from build123d import *

# Parameters (mm, degrees)
SKETCH1_W                                       = 75
SKETCH1_H                                       = 108
BOSS_EXTRUDE1_DEPTH                             = 10
SKETCH2_R                                       = 6
SKETCH2_R_2                                     = 5
CUT_EXTRUDE2_DEPTH                              = 115.761709642
HOLE_WIZARD_M31_D                               = 3.2
HOLE_WIZARD_M31_CSINK_D                         = 6.3
HOLE_WIZARD_M31_CSINK_ANGLE                     = 90
BOSS_EXTRUDE2_DEPTH                             = 75
BOSS_EXTRUDE3_DEPTH                             = 7
CHAMFER2_SIZE                                   = 0.5
HOLE_WIZARD_M41_DEPTH                           = 10
CHAMFER4_SIZE                                   = 0.5
CUT_EXTRUDE3_DEPTH                              = 122.762603454
CSK_FOR_M2_FLAT_HEAD_MACHINE_SCREW1_D           = 2.2
CSK_FOR_M2_FLAT_HEAD_MACHINE_SCREW1_CSINK_D     = 4.4
CSK_FOR_M2_FLAT_HEAD_MACHINE_SCREW1_CSINK_ANGLE = 90
M5X0_8_TAPPED_HOLE1_D                           = 4.2
M5X0_8_TAPPED_HOLE1_DEPTH                       = 10.4
M5X0_8_TAPPED_HOLE1_TIP                         = 1.2618073
CHAMFER6_SIZE                                   = 10


with BuildPart() as part:
    # Sketch1 → Boss-Extrude1 (new body)
    with BuildSketch(Plane.XY):
        with Locations((0, -54)):
            Rectangle(SKETCH1_W, SKETCH1_H)
    extrude(amount=BOSS_EXTRUDE1_DEPTH)

    # Sketch2 → Cut-Extrude2 (cut, through all)
    with BuildSketch(Plane.XY):
        with Locations((16, -25)):
            Circle(SKETCH2_R)
        with Locations((-17, -25)):
            Circle(SKETCH2_R_2)
    extrude(amount=CUT_EXTRUDE2_DEPTH, mode=Mode.SUBTRACT)

    # Зенковка для  винта с плоской головкой M31 (through all)
    with Locations(Plane.XY.offset(10)):
        with Locations((26.825317547, -18.75), (5.174682453, -18.75), (5.174682453, -31.25), (26.825317547, -31.25)):
            CounterSinkHole(HOLE_WIZARD_M31_D / 2, HOLE_WIZARD_M31_CSINK_D / 2, counter_sink_angle=HOLE_WIZARD_M31_CSINK_ANGLE)

    # Sketch13 → Boss-Extrude2 (add, through all)
    with BuildSketch(Plane(origin=(37.5, 0, 0), x_dir=(0, 0, -1), z_dir=(1, 0, 0))):
        Polygon((-10, -97.69), (-13.96, -101.65), (-13.96, -108), (-10, -108), (0, -108), (3.96, -108), (3.96, -101.65), (0, -97.69), align=None)
    extrude(amount=-BOSS_EXTRUDE2_DEPTH)

    # Sketch14 → Boss-Extrude3 (add)
    with BuildSketch(Plane.XZ.offset(108)):
        with BuildLine():
            Line((-2.5, 0), (-2.5, 10))
            ThreePointArc((-2.5, 10), (0, 12.5), (2.5, 10))
            Line((2.5, 10), (2.5, 0))
            ThreePointArc((2.5, 0), (0, -2.5), (-2.5, 0))
        make_face()
        with BuildLine():
            Line((22.5, 0), (22.5, 10))
            ThreePointArc((22.5, 10), (25, 12.5), (27.5, 10))
            Line((27.5, 10), (27.5, 0))
            ThreePointArc((27.5, 0), (25, -2.5), (22.5, 0))
        make_face()
        with BuildLine():
            Line((-27.5, 0), (-27.5, 10))
            ThreePointArc((-27.5, 10), (-25, 12.5), (-22.5, 10))
            Line((-22.5, 10), (-22.5, 0))
            ThreePointArc((-22.5, 0), (-25, -2.5), (-27.5, 0))
        make_face()
    extrude(amount=BOSS_EXTRUDE3_DEPTH)

    # Chamfer2
    chamfer2_edges = [part.edges().sort_by_distance(p)[0] for p in [
        (-25, -115, 12.5),
        (-27.5, -115, 5),
        (-25, -115, -2.5),
        (-22.5, -115, 5),
        (0, -115, 12.5),
        (-2.5, -115, 5),
        (0, -115, -2.5),
        (2.5, -115, 5),
        (25, -115, 12.5),
        (22.5, -115, 5),
        (25, -115, -2.5),
        (27.5, -115, 5),
    ]]
    chamfer(chamfer2_edges, length=CHAMFER2_SIZE)

    # Зенковка для  винта с потайной головкой с внутренним шестигранником M41: read off the stored shape, not the designer's step
    # Зенковка для  винта с потайной головкой с внутренним шестигранником M41 outline → Зенковка для  винта с потайной головкой с внутренним шестигранником M41 (cut)
    with BuildSketch(Plane.XY):
        with BuildLine():
            Line((13.75, -36.25), (13.75, -38.75))
            ThreePointArc((13.75, -38.75), (16, -41), (18.25, -38.75))
            Line((18.25, -38.75), (18.25, -36.25))
            ThreePointArc((18.25, -36.25), (16, -34), (13.75, -36.25))
        make_face()
        with BuildLine():
            Line((18.25, -13.75), (18.25, -11.25))
            ThreePointArc((18.25, -11.25), (16, -9), (13.75, -11.25))
            Line((13.75, -11.25), (13.75, -13.75))
            ThreePointArc((13.75, -13.75), (16, -16), (18.25, -13.75))
        make_face()
    extrude(amount=HOLE_WIZARD_M41_DEPTH, mode=Mode.SUBTRACT)

    # Hole Wizard M41 2: loft between two sections, ruled curve by curve
    hole_wizard_m41_2_from = [
        Edge.make_three_point_arc((13.75, -38.75, 7.77), (14.409009742, -40.340990258, 7.77), (16, -41, 7.77)),
        Edge.make_three_point_arc((16, -41, 7.77), (17.590990258, -40.340990258, 7.77), (18.25, -38.75, 7.77)),
        Edge.make_three_point_arc((18.25, -36.25, 7.77), (17.590990258, -34.659009742, 7.77), (16, -34, 7.77)),
        Edge.make_three_point_arc((16, -34, 7.77), (14.409009742, -34.659009742, 7.77), (13.75, -36.25, 7.77)),
        Edge.make_line((18.25, -38.75, 7.77), (18.25, -36.25, 7.77)),
        Edge.make_line((13.75, -38.75, 7.77), (13.75, -36.25, 7.77)),
    ]
    hole_wizard_m41_2_to = [
        Edge.make_three_point_arc((11.52, -38.75, 10), (12.83216162, -41.91783838, 10), (16, -43.23, 10)),
        Edge.make_three_point_arc((16, -43.23, 10), (19.16783838, -41.91783838, 10), (20.48, -38.75, 10)),
        Edge.make_three_point_arc((20.48, -36.25, 10), (19.16783838, -33.08216162, 10), (16, -31.77, 10)),
        Edge.make_three_point_arc((16, -31.77, 10), (12.83216162, -33.08216162, 10), (11.52, -36.25, 10)),
        Edge.make_line((20.48, -38.75, 10), (20.48, -36.25, 10)),
        Edge.make_line((11.52, -38.75, 10), (11.52, -36.25, 10)),
    ]
    hole_wizard_m41_2 = Solid(Shell([*[Face.make_surface_from_curves(hole_wizard_m41_2_from[k], hole_wizard_m41_2_to[k]) for k in range(6)], Face(Wire(hole_wizard_m41_2_from)), Face(Wire(hole_wizard_m41_2_to))]))
    add(hole_wizard_m41_2, mode=Mode.SUBTRACT)

    # Hole Wizard M41 3: loft between two sections, ruled curve by curve
    hole_wizard_m41_3_from = [
        Edge.make_three_point_arc((13.75, -13.75, 7.77), (14.409009742, -15.340990258, 7.77), (16, -16, 7.77)),
        Edge.make_three_point_arc((16, -16, 7.77), (17.590990258, -15.340990258, 7.77), (18.25, -13.75, 7.77)),
        Edge.make_three_point_arc((18.25, -11.25, 7.77), (17.590990258, -9.659009742, 7.77), (16, -9, 7.77)),
        Edge.make_three_point_arc((16, -9, 7.77), (14.409009742, -9.659009742, 7.77), (13.75, -11.25, 7.77)),
        Edge.make_line((18.25, -13.75, 7.77), (18.25, -11.25, 7.77)),
        Edge.make_line((13.75, -13.75, 7.77), (13.75, -11.25, 7.77)),
    ]
    hole_wizard_m41_3_to = [
        Edge.make_three_point_arc((11.52, -13.75, 10), (12.83216162, -16.91783838, 10), (16, -18.23, 10)),
        Edge.make_three_point_arc((16, -18.23, 10), (19.16783838, -16.91783838, 10), (20.48, -13.75, 10)),
        Edge.make_three_point_arc((20.48, -11.25, 10), (19.16783838, -8.08216162, 10), (16, -6.77, 10)),
        Edge.make_three_point_arc((16, -6.77, 10), (12.83216162, -8.08216162, 10), (11.52, -11.25, 10)),
        Edge.make_line((20.48, -13.75, 10), (20.48, -11.25, 10)),
        Edge.make_line((11.52, -13.75, 10), (11.52, -11.25, 10)),
    ]
    hole_wizard_m41_3 = Solid(Shell([*[Face.make_surface_from_curves(hole_wizard_m41_3_from[k], hole_wizard_m41_3_to[k]) for k in range(6)], Face(Wire(hole_wizard_m41_3_from)), Face(Wire(hole_wizard_m41_3_to))]))
    add(hole_wizard_m41_3, mode=Mode.SUBTRACT)

    # Chamfer4
    chamfer4_edges = [part.edges().sort_by_distance(p)[0] for p in [
        (10, -25, 0),
        (10, -25, 10),
        (13.75, -37.5, 0),
        (16, -41, 0),
        (16, -34, 0),
        (18.25, -37.5, 0),
        (16, -9, 0),
        (18.25, -12.5, 0),
        (13.75, -12.5, 0),
        (16, -16, 0),
        (-22, -25, 0),
        (-22, -25, 10),
        (28.425317547, -31.25, 0),
        (6.774682453, -31.25, 0),
        (6.774682453, -18.75, 0),
        (28.425317547, -18.75, 0),
    ]]
    chamfer(chamfer4_edges, length=CHAMFER4_SIZE)

    # Sketch22 → Cut-Extrude3 (cut, through all)
    with BuildSketch(Plane.XY.offset(10)):
        with BuildLine():
            Line((2.5, -96.69), (-2.5, -96.69))
            ThreePointArc((-2.5, -96.69), (-6.035533906, -95.225533906), (-7.5, -91.69))
            Line((-7.5, -91.69), (-7.5, -57.69))
            ThreePointArc((-7.5, -57.69), (-6.035533906, -54.154466094), (-2.5, -52.69))
            Line((-2.5, -52.69), (2.5, -52.69))
            ThreePointArc((2.5, -52.69), (6.035533906, -54.154466094), (7.5, -57.69))
            Line((7.5, -57.69), (7.5, -91.69))
            ThreePointArc((7.5, -91.69), (6.035533906, -95.225533906), (2.5, -96.69))
        make_face()
        with BuildLine():
            Line((-22.5, -96.69), (-27.5, -96.69))
            ThreePointArc((-27.5, -96.69), (-31.035533906, -95.225533906), (-32.5, -91.69))
            Line((-32.5, -91.69), (-32.5, -57.69))
            ThreePointArc((-32.5, -57.69), (-31.035533906, -54.154466094), (-27.5, -52.69))
            Line((-27.5, -52.69), (-22.5, -52.69))
            ThreePointArc((-22.5, -52.69), (-18.964466094, -54.154466094), (-17.5, -57.69))
            Line((-17.5, -57.69), (-17.5, -91.69))
            ThreePointArc((-17.5, -91.69), (-18.964466094, -95.225533906), (-22.5, -96.69))
        make_face()
        with BuildLine():
            Line((27.5, -96.69), (22.5, -96.69))
            ThreePointArc((22.5, -96.69), (18.964466094, -95.225533906), (17.5, -91.69))
            Line((17.5, -91.69), (17.5, -57.69))
            ThreePointArc((17.5, -57.69), (18.964466094, -54.154466094), (22.5, -52.69))
            Line((22.5, -52.69), (27.5, -52.69))
            ThreePointArc((27.5, -52.69), (31.035533906, -54.154466094), (32.5, -57.69))
            Line((32.5, -57.69), (32.5, -91.69))
            ThreePointArc((32.5, -91.69), (31.035533906, -95.225533906), (27.5, -96.69))
        make_face()
    extrude(amount=-CUT_EXTRUDE3_DEPTH, mode=Mode.SUBTRACT)

    # CSK for M2 Flat Head Machine Screw1 (through all)
    with Locations(Plane.XY.offset(10)):
        with Locations((-17, -17.5), (-17, -32.5)):
            CounterSinkHole(CSK_FOR_M2_FLAT_HEAD_MACHINE_SCREW1_D / 2, CSK_FOR_M2_FLAT_HEAD_MACHINE_SCREW1_CSINK_D / 2, counter_sink_angle=CSK_FOR_M2_FLAT_HEAD_MACHINE_SCREW1_CSINK_ANGLE)

    # M5x0.8 Tapped Hole1
    with Locations(Plane(origin=(0, -108, 0), x_dir=(-1, 0, 0), z_dir=(0, -1, 0))):
        with Locations((32.5, -5), (13.75, -5), (-13.75, -5), (-32.5, -5)):
            Hole(M5X0_8_TAPPED_HOLE1_D / 2, depth=M5X0_8_TAPPED_HOLE1_DEPTH)
            with Locations((0, 0, -(M5X0_8_TAPPED_HOLE1_DEPTH + M5X0_8_TAPPED_HOLE1_TIP / 2))):  # 118° drill point
                Cone(0, M5X0_8_TAPPED_HOLE1_D / 2, M5X0_8_TAPPED_HOLE1_TIP, mode=Mode.SUBTRACT)

    # Chamfer6
    chamfer6_edges = [part.edges().sort_by_distance(p)[0] for p in [
        (-37.5, 0, 5),
        (37.5, 0, 5),
    ]]
    chamfer(chamfer6_edges, length=CHAMFER6_SIZE)


solid = part.part
Input: part model. Units: mm. Frame: model coordinates. A direction names the side the tool comes from. Coordinates: 2 decimals unless noted, no trailing zeros. Write each loop counter-clockwise with the first axis right and the second up, starting at its lowest first coordinate (ties: lowest second). Pieces come first, ordered by that corner, then holes. Notation, with made-up numbers: M -27.75,-9 L 20.25,-9 A23 cw 20.25,17 Z; hole C 8.5,52.25 d4. An arc over 180 degrees is marked long. Answer as a JSON object with one key per item and string values. Group by question number.
(1) Contact query for flat-ended pins moving along their axis: P1, Ø3.5, axis at x = -13.75, z = 5, coming from the -Y side; P2, Ø2.5, axis at x = -32.5, z = 5, coming from the -Y side; P3, Ø22.5, axis at x = -7.5, y = -31.5, coming from the -Z side. Output: stop coordinate, or through.
(2) Ray query, line 1 along X through (y, z) = (-25, 5.75); line 2 along X through (y, z) = (-92, 4.75); line 3 along Y through (x, z) = (16, 5.75). Return the intervals inside material, ascending. Write a range as [from, to].
(3) Section C-C on y = -87.5. Output: boundary loops of the cut face in (x, z), plus the area to 3 significant figures.
(4) Mould query, pull axis Y, two halves, no side actions, for faces 1 (the face through (17.5, -75, 5)), 2 (the face through (-27.5, -111, 5)), 3 (the face through (19, -95.26, 5.07)), 4 (the face through (-24.953, -114.865, -2.135)). Classes: pulls with the +Y half, pulls with the -Y half, needs draft (parallel to the pull), parting line crosses it, or undercut.
(5) Section B-B on x = 0. Output: boundary loops of the cut face in (y, z).
(6) Section A-A on y = -25. Output: boundary loops of the cut face in (x, z), plus the area to 3 significant figures.
(7) Set-up query: faces 5 (the face through (1, -105, -3.96)), 6 (the face through (-1, -48, 10)), 7 (the face through (25, -52.69, 5)), 8 (the face through (24.9, -111.2, 12.5)). Return all of +Z, -Z, +X, -X, +Y, -Y with unobstructed straight access to the full face (end or side cutting, diameter ignored); none if empty.
Result set:
{
 "1": {"P1": "stops at y = -97.39", "P2": "stops at y = -97.09", "P3": "stops at z = 0"},
 "2": {"line 1": "x = [-37.5, -22], [-12, 10], [22, 37.5]", "line 2": "x = [-37.5, -32.49], [-17.51, -7.49], [7.49, 17.51], [32.49, 37.5]", "line 3": "y = [-108, -41], [-34, -31], [-19, -16], [-9, 0]"},
 "3": {"outline": "M -37.5,0 L -32.5,0 L -32.5,10 L -37.5,10 Z; M -17.5,0 L -7.5,0 L -7.5,10 L -17.5,10 Z; M 7.5,0 L 17.5,0 L 17.5,10 L 7.5,10 Z; M 32.5,0 L 37.5,0 L 37.5,10 L 32.5,10 Z", "area": "300 mm2"},
 "4": {"face 1": "undercut", "face 2": "needs draft", "face 3": "undercut", "face 4": "pulls with the -Y half"},
 "5": {"outline": "M -115,-2 L -114.5,-2.5 L -108,-2.5 L -108,-3.96 L -101.65,-3.96 L -97.69,0 L -96.69,0 L -96.69,10 L -97.69,10 L -101.65,13.96 L -108,13.96 L -108,12.5 L -114.5,12.5 L -115,12 Z; M -52.69,0 L 0,0 L 0,10 L -52.69,10 Z"},
 "6": {"outline": "M -37.5,0 L -22.5,0 L -22,0.5 L -22,9.5 L -22.5,10 L -37.5,10 Z; M -12,0.5 L -11.5,0 L 9.5,0 L 10,0.5 L 10,9.5 L 9.5,10 L -11.5,10 L -12,9.5 Z; M 22,0.5 L 22.5,0 L 37.5,0 L 37.5,10 L 22.5,10 L 22,9.5 Z", "area": "529 mm2"},
 "7": {"face 5": "-Z, +X, -X, +Y, -Y", "face 6": "+Z, +X, -X, +Y", "face 7": "+Z, -Z", "face 8": "+Z, -Y"}
}
